Here's how the part is built. I have some questions about the finished solid (model axes, mm). A direction names the side the tool comes from. Round coordinates to 2 decimals unless told otherwise and drop trailing zeros. Loops run counter-clockwise (first coordinate to the right, second up) from the corner with the lowest first, then second, coordinate; pieces in that order, holes last. Notation, with made-up numbers: M -19,79.5 L -4,79.5 A21 ccw -4,93.5 Z; hole C -34.5,23 d9. An arc over 180 degrees is marked long. Use a Markdown table: item, result.
from build123d import *

# Parameters (mm, degrees)
EXTRU_MINCE2_DEPTH      = 200
EPAISSIR5_DEPTH         = 200
EPAISSIR7_DEPTH         = 200
EXTRU_MINCE3_DEPTH      = 20
EXTRU_MINCE3_DEPTH_BACK = 15


# Read off the part's stored shape, not the designer's step: Epaissir5, Epaissir7
with BuildPart() as part:
    # Esquisse3 → Extru.-Mince2 (new body)
    with BuildSketch(Plane.XY):
        with BuildLine():
            Line((-206.649507199, -11.92714811), (-206.649507199, -3.47401752))
            Line((-206.649507199, -3.47401752), (-206.649507199, 81.52598248))
            ThreePointArc((-206.649507199, 81.52598248), (-196.691137759, 105.56761304), (-172.649507199, 115.52598248))
            Line((-172.649507199, 115.52598248), (-82.649507199, 115.52598248))
            ThreePointArc((-82.649507199, 115.52598248), (-58.607876638, 105.56761304), (-48.649507199, 81.52598248))
            Line((-48.649507199, 81.52598248), (-48.649507199, -11.92714811))
            ThreePointArc((-48.649507199, -11.92714811), (-61.399009455, -38.338842544), (-78.173060849, -62.396244951))
            ThreePointArc((-78.173060849, -62.396244951), (-102.275198337, -78.711501116), (-127.649507199, -92.967905467))
            ThreePointArc((-127.649507199, -92.967905467), (-153.023816061, -78.711501116), (-177.125953549, -62.396244951))
            ThreePointArc((-177.125953549, -62.396244951), (-193.900004942, -38.338842544), (-206.649507199, -11.92714811))
        make_face()
        with BuildLine():
            Line((-202.649507199, -11.17401752), (-202.649507199, -3.47401752))
            Line((-202.649507199, -3.47401752), (-202.649507199, 81.52598248))
            ThreePointArc((-202.649507199, 81.52598248), (-193.862710634, 102.739185916), (-172.649507199, 111.52598248))
            Line((-172.649507199, 111.52598248), (-82.649507199, 111.52598248))
            ThreePointArc((-82.649507199, 111.52598248), (-61.436303763, 102.739185916), (-52.649507199, 81.52598248))
            Line((-52.649507199, 81.52598248), (-52.649507199, -11.17401752))
            ThreePointArc((-52.649507199, -11.17401752), (-64.915375774, -36.427970301), (-80.949507199, -59.47401752))
            ThreePointArc((-80.949507199, -59.47401752), (-103.722688687, -74.902894226), (-127.649507199, -88.47401752))
            ThreePointArc((-127.649507199, -88.47401752), (-151.57632571, -74.902894226), (-174.349507199, -59.47401752))
            ThreePointArc((-174.349507199, -59.47401752), (-190.383638623, -36.427970301), (-202.649507199, -11.17401752))
        make_face(mode=Mode.SUBTRACT)
    extrude(amount=EXTRU_MINCE2_DEPTH)

    # Epaissir5 outline → Epaissir5 (add)
    with BuildSketch(Plane.XY):
        with BuildLine():
            add(Edge.make_bspline(
                [(-78.173060849, -62.396244951), (-91.313583381, -75.858349648), (-107.794638855, -86.055391974), (-127.649507199, -92.967905467)],
                knots=[0.501331546, 0.501331546, 0.501331546, 0.501331546, 1, 1, 1, 1], degree=3))
            ThreePointArc((-78.173060849, -62.396244951), (-102.275198337, -78.711501116), (-127.649507199, -92.967905467))
        make_face()
        with BuildLine():
            add(Edge.make_bspline(
                [(-48.649507199, -11.92714811), (-55.127972189, -32.028220402), (-64.962362616, -48.862247174), (-78.173060849, -62.396244951)],
                knots=[0, 0, 0, 0, 0.501331546, 0.501331546, 0.501331546, 0.501331546], degree=3))
            ThreePointArc((-48.649507199, -11.92714811), (-61.399009455, -38.338842545), (-78.173060849, -62.396244951))
        make_face()
    extrude(amount=EPAISSIR5_DEPTH)

    # Epaissir7 outline → Epaissir7 (add)
    with BuildSketch(Plane.XY):
        with BuildLine():
            ThreePointArc((-177.125953549, -62.396244951), (-193.900004942, -38.338842544), (-206.649507199, -11.92714811))
            add(Edge.make_bspline(
                [(-206.649507199, -11.92714811), (-200.171042209, -32.028220402), (-190.336651781, -48.862247174), (-177.125953549, -62.396244951)],
                knots=[0, 0, 0, 0, 0.501331546, 0.501331546, 0.501331546, 0.501331546], degree=3))
        make_face()
        with BuildLine():
            ThreePointArc((-127.649507199, -92.967905467), (-153.023816061, -78.711501116), (-177.125953549, -62.396244951))
            add(Edge.make_bspline(
                [(-177.125953549, -62.396244951), (-163.985431016, -75.858349648), (-147.504375542, -86.055391974), (-127.649507199, -92.967905467)],
                knots=[0.501331546, 0.501331546, 0.501331546, 0.501331546, 1, 1, 1, 1], degree=3))
        make_face()
    extrude(amount=EPAISSIR7_DEPTH)

    # Esquisse7 → Extru.-Mince3 (add, two sides: drawn at the far end of the back side and taken through both)
    with BuildSketch(Plane.XY.offset(200).offset(-EXTRU_MINCE3_DEPTH_BACK)):
        with BuildLine():
            Line((-202.649507199, -11.17401752), (-202.649507199, -3.47401752))
            Line((-202.649507199, -3.47401752), (-202.649507199, 81.52598248))
            ThreePointArc((-202.649507199, 81.52598248), (-193.862710634, 102.739185916), (-172.649507199, 111.52598248))
            Line((-172.649507199, 111.52598248), (-82.649507199, 111.52598248))
            ThreePointArc((-82.649507199, 111.52598248), (-61.436303763, 102.739185916), (-52.649507199, 81.52598248))
            Line((-52.649507199, 81.52598248), (-52.649507199, -11.17401752))
            ThreePointArc((-52.649507199, -11.17401752), (-64.915375774, -36.427970301), (-80.949507199, -59.47401752))
            ThreePointArc((-80.949507199, -59.47401752), (-103.722688687, -74.902894226), (-127.649507199, -88.47401752))
            ThreePointArc((-127.649507199, -88.47401752), (-151.57632571, -74.902894226), (-174.349507199, -59.47401752))
            ThreePointArc((-174.349507199, -59.47401752), (-190.383638623, -36.427970301), (-202.649507199, -11.17401752))
        make_face()
        with BuildLine():
            Line((-200.649507199, -10.794210022), (-200.649507199, -3.47401752))
            Line((-200.649507199, -3.47401752), (-200.649507199, 81.52598248))
            ThreePointArc((-200.649507199, 81.52598248), (-192.448497072, 101.324972353), (-172.649507199, 109.52598248))
            Line((-172.649507199, 109.52598248), (-82.649507199, 109.52598248))
            ThreePointArc((-82.649507199, 109.52598248), (-62.850517326, 101.324972353), (-54.649507199, 81.52598248))
            Line((-54.649507199, 81.52598248), (-54.649507199, -10.794210022))
            ThreePointArc((-54.649507199, -10.794210022), (-66.673062941, -35.471620796), (-82.338728425, -58.013302636))
            ThreePointArc((-82.338728425, -58.013302636), (-104.44621972, -72.997686116), (-127.649507199, -86.221920301))
            ThreePointArc((-127.649507199, -86.221920301), (-150.852794678, -72.997686116), (-172.960285972, -58.013302636))
            ThreePointArc((-172.960285972, -58.013302636), (-188.625951457, -35.471620796), (-200.649507199, -10.794210022))
        make_face(mode=Mode.SUBTRACT)
    extrude(amount=EXTRU_MINCE3_DEPTH + EXTRU_MINCE3_DEPTH_BACK)


solid = part.part
1. We'd pull the mould along X, two halves only. Please class faces 5 (the face through (-150.535, -73.195, 202.255)), 6 (the face through (-190.184, -36.767, 209.86)), 7 (the face through (-128, 111.526, 210)): +X half, -X half, draft (parallel to the pull), parting line (faces both ways), or undercut.
Answer sheet:
| item | result |
|---|---|
| face 5 | undercut |
| face 6 | -X half |
| face 7 | draft |
2. Imagine slicing it at B-B, the plane y = 85.5. Write out the boundary of the cut face in (x, z), then the cut area to 3 significant figures.
Answer sheet:
| item | result |
|---|---|
| outline | M -206.42,0 L -202.39,0 L -202.39,185 L -200.37,185 L -200.37,220 L -202.39,220 L -202.39,200 L -206.42,200 Z; M -54.93,185 L -52.91,185 L -52.91,0 L -48.88,0 L -48.88,200 L -52.91,200 L -52.91,220 L -54.93,220 Z |
| area | 1,750 mm2 |
3. Which directions (+Z, -Z, +X, -X, +Y, -Y) give clear straight access to the entire face, cutting with the end or side of a thin tool? Please do faces 1 (the face through (-66.48, -35.14, 202.26)), 2 (the face through (-202.65, 35, 91)), 3 (the face through (-194.1, 102.5, 209.9)), 4 (the face through (-202.65, 35, 210)).
Answer sheet:
| item | result |
|---|---|
| face 1 | +Z, -Z |
| face 2 | -Z |
| face 3 | +Z, -X, +Y |
| face 4 | +Z, -X, +Y, -Y |
4. Imagine slicing it at A-A, the plane y = 12. Write out the boundary of the cut face in (x, z), then the cut area to 3 significant figures.
Answer sheet:
| item | result |
|---|---|
| outline | M -206.65,0 L -202.65,0 L -202.65,185 L -200.65,185 L -200.65,220 L -202.65,220 L -202.65,200 L -206.65,200 Z; M -54.65,185 L -52.65,185 L -52.65,0 L -48.65,0 L -48.65,200 L -52.65,200 L -52.65,220 L -54.65,220 Z |
| area | 1,740 mm2 |
5. For pin 1 Ø8 at (x, z) = (-175, 161.5) entering from -Y; pin 2 Ø22 at (y, z) = (30, 213.5) entering from -X; pin 3 Ø10 at (y, z) = (-65, 64) entering from -X, each with a flat end and sliding along its axis, tell me the tip position at first contact or that it passes through.
Answer sheet:
| item | result |
|---|---|
| pin 1 | y = -68.22 |
| pin 2 | x = -202.65 |
| pin 3 | x = -179.4 |
6. I need wall thicknesses on probe 1 along X at (y, z) = (38.5, 44); probe 2 along Z at (x, y) = (-165, -67.5); probe 3 along Y at (x, z) = (-153.5, 143). Which ranges of each line are inside material? Lowest first, please. Write a range as from..to.
Answer sheet:
| item | result |
|---|---|
| probe 1 | -206.65..-202.65, -52.65..-48.65 |
| probe 2 | 0..200 |
| probe 3 | -80.99..-73.7, 111.53..115.53 |
